Part print with two shaded views. Sizes in mm from the minimum x, y, z corner. Round coordinates to 2 decimals unless told otherwise and drop trailing zeros. Loops run counter-clockwise (first coordinate to the right, second up) from the corner with the lowest first, then second, coordinate; pieces in that order, holes last. Notation, with made-up numbers: (9, -8.5) -> (13, -8.5) arc R18 ccw to (13, 4.5) -> close; hole circle Ø9 at (59, 44.25). An arc over 180 degrees is marked (long way). Use a Markdown table: item, result. Add a question column.
Item 1: Cut at C-C, the plane z = 6.5. List the corners of the cut face in (x, y).
Item 2: Cut at A-A, the plane x = 10. List the corners of the cut face in (y, z), plus the area to 3 significant figures.
Item 3: Cut at D-D, the plane x = 2.25. List the corners of the cut face in (y, z), plus the area to 3 significant figures.
Item 4: Two-plate mould, pull along Y, no slides. Class the marked faces 1 and 2: pulls with the +Y half, pulls with the -Y half, needs draft (parallel to the pull), parting line crosses it, or undercut.
Item 5: Flat gauge pins, fed straight in: pin 1 (8 mm diameter, centred on x = 4, z = 2.5, fed in from +Y); pin 2 (1 mm diameter, centred on x = 6.5, z = 8, fed in from +Y); pin 3 (1 mm diameter, centred on x = 15.5, z = 10, fed in from +Y). Where does each tip first touch, or does it go through?
Item 6: Probe line 1 (Y direction, x = 10, z = 14.85); line 2 (Z direction, x = 12, y = 4.5); line 3 (Y direction, x = 13.5, z = 0.5). List the from-to ranges inside material, lowest first. Write a range as [from, to].
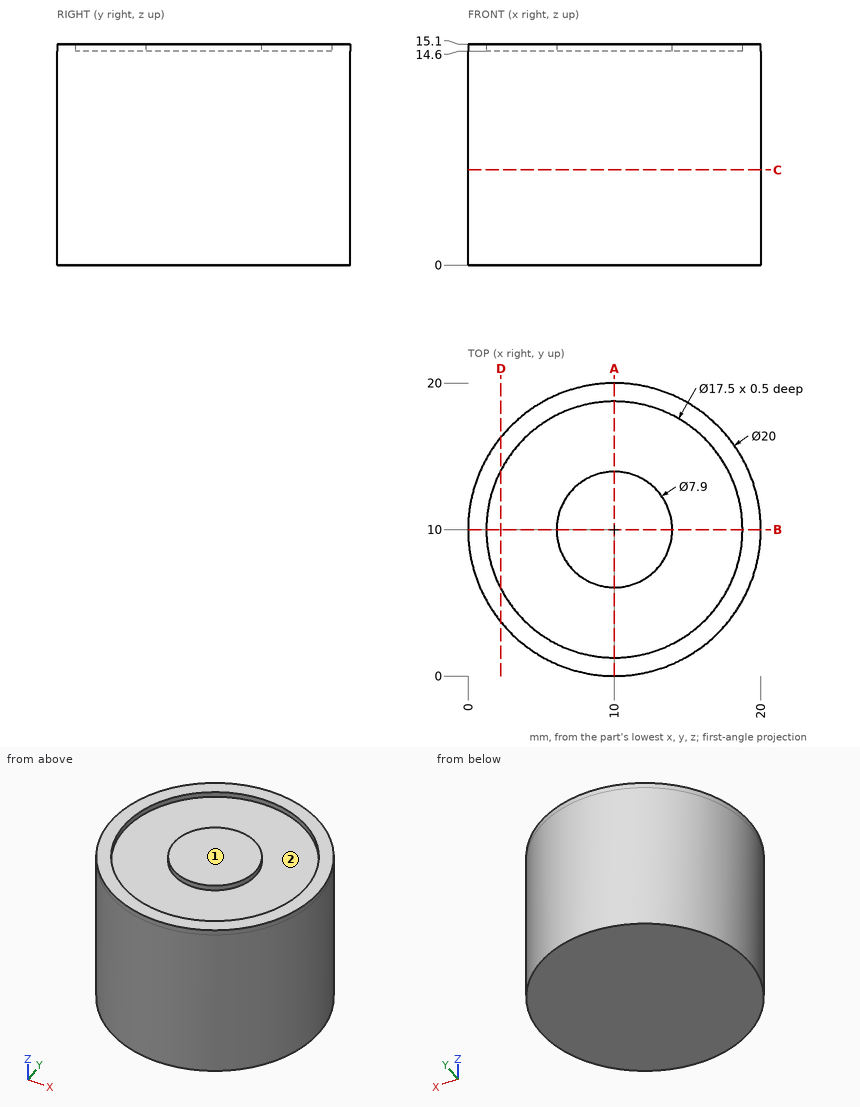
A:
| question | item | result |
|---|---|---|
| 1 | outline | circle Ø20 at (10, 10) |
| 2 | outline | (0, 0) -> (20, 0) -> (20, 15.1) -> (18.75, 15.1) -> (18.75, 14.6) -> (13.95, 14.6) -> (13.95, 15.1) -> (6.05, 15.1) -> (6.05, 14.6) -> (1.25, 14.6) -> (1.25, 15.1) -> (0, 15.1) -> close |
| 2 | area | 297 mm^2 |
| 3 | outline | (3.68, 0) -> (16.32, 0) -> (16.32, 15.1) -> (14.06, 15.1) -> (14.06, 14.6) -> (5.94, 14.6) -> (5.94, 15.1) -> (3.68, 15.1) -> close |
| 3 | area | 187 mm^2 |
| 4 | face 1 | needs draft |
| 4 | face 2 | undercut |
| 5 | pin 1 | stops at y = 19.8 |
| 5 | pin 2 | stops at y = 19.54 |
| 5 | pin 3 | stops at y = 18.66 |
| 6 | line 1 | y = [0, 1.25], [6.05, 13.95], [18.75, 20] |
| 6 | line 2 | z = [0, 14.6] |
| 6 | line 3 | y = [0.63, 19.37] |
